Work out the finished part from the listing and answer in its coordinate system (mm). Face numbers are marked on the shaded views. Round coordinates to 2 decimals unless told otherwise and drop trailing zeros. Loops run counter-clockwise (first coordinate to the right, second up) from the corner with the lowest first, then second, coordinate; pieces in that order, holes last. Notation, with made-up numbers: (28, 37.5) - (84, 37.5) arc R28 cw to (84, 68.5) - close; hole circle Ø5 at (37.25, 47). An arc over 180 degrees is marked (long way). Return JSON: item names as keys, results as strings.
from build123d import *

# Parameters (mm, degrees)
F0_R      = 49.071094
F1_DEPTH  = 400
F2_R      = 45.183213
F3_DEPTH  = 408.94
F3_FACE_R = 45.183213
F4_DEPTH  = 500.38


with BuildPart() as f1:
    # F0 (on Front) → F1 (new body)
    with BuildSketch(Plane.XZ):
        Circle(F0_R)
    extrude(amount=-F1_DEPTH)

    # F2 (on face) → F3 (join)
    with BuildSketch(Plane(origin=(0, 400, 0), x_dir=(-1, 0, 0), z_dir=(0, 1, 0))):
        Circle(F2_R)
    extrude(amount=-F3_DEPTH)

    # F3_face (on face) → F4 (cut)
    with BuildSketch(Plane(origin=(0, -8.94, 0), x_dir=(-1, 0, 0), z_dir=(0, -1, 0))):
        Circle(F3_FACE_R)
    extrude(amount=-F4_DEPTH, mode=Mode.SUBTRACT)


solid = f1.part
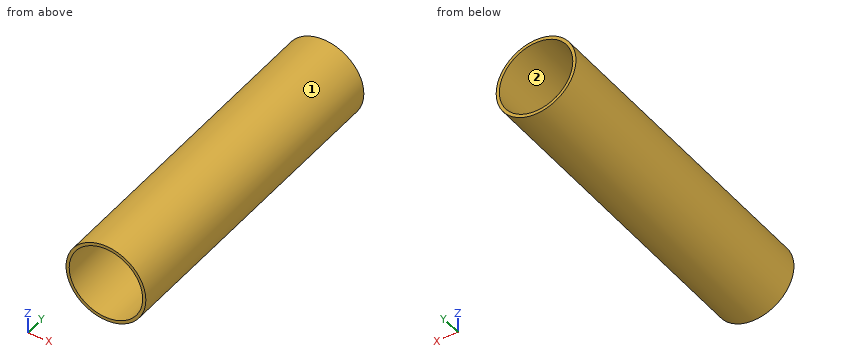
1) Section B-B (z = 0) is taken. Give the vertices of the cut face in (x, y).
Verdict:
{"outline": "(-49.07, 0) - (-45.18, 0) - (-45.18, 400) - (-49.07, 400) - close; (45.18, 0) - (49.07, 0) - (49.07, 400) - (45.18, 400) - close"}
2) Section C-C (y = 122.5) is taken. Give the vertices of the cut face in (x, z), and give its area (3 significant figures).
Verdict:
{"outline": "circle Ø98.14 at (0, 0); hole circle Ø90.37 at (0, 0)", "area": "1,150 mm2"}
3) Find the intervals of material crossed by L1, parallel to Z at x = 0, y = 200.5; L2, parallel to Z at x = -2, y = 64; L3, parallel to X at y = 252, z = -20, in increasing order.
Verdict:
{"L1": "z = -49.07 to -45.18, 45.18 to 49.07", "L2": "z = -49.03 to -45.14, 45.14 to 49.03", "L3": "x = -44.81 to -40.52, 40.52 to 44.81"}
4) Determine the mould class of the marked faces 1 and 2 for opening direction Z: pulls with the +Z half, pulls with the -Z half, needs draft (parallel to the pull), parting line crosses it, or undercut.
Verdict:
{"face 1": "parting line crosses it", "face 2": "undercut"}
5) Flat-ended cylindrical pins translate along their axes: pin 1 (12 mm diameter, centred on y = 310.5, z = -13.5, fed in from -X); pin 2 (1 mm diameter, centred on y = 58.5, z = -29.5, fed in from +X) (3 decimals); pin 3 (2 mm diameter, centred on x = -32, z = -39, fed in from -Y); pin 4 (12 mm diameter, centred on y = 96, z = -37.5, fed in from +X). Find the tip coordinate at first contact, or state that the pin passes through.
Verdict:
{"pin 1": "stops at x = -48.49", "pin 2": "stops at x = 39.585", "pin 3": "passes through", "pin 4": "stops at x = 37.63"}
6) Section A-A (x = 0) is taken. Give the vertices of the cut face in (y, z).
Verdict:
{"outline": "(0, -49.07) - (400, -49.07) - (400, -45.18) - (0, -45.18) - close; (0, 45.18) - (400, 45.18) - (400, 49.07) - (0, 49.07) - close"}
